Design review of the part built by this model. Coordinates are the model's own, in mm. Give positions to 0.01 mm unless a question says otherwise; leave off trailing zeros. Loops run counter-clockwise (first coordinate to the right, second up) from the corner with the lowest first, then second, coordinate; pieces in that order, holes last. Notation, with made-up numbers: (47, 82) -> (64, 82) arc R24 ccw to (64, 108) -> close; hole circle Ø1 at (62, 8.5). An arc over 180 degrees is marked (long way). Use CSV: the item, a comma, the result in double quotes. Start each with the question number.
Item 1: Clearance check with flat-ended pins moving along their axes: pin 1 (1.5 mm diameter, centred on x = 63.5, z = 22.5, fed in from -Y); pin 2 (1.5 mm diameter, centred on x = 85.5, y = 2, fed in from -Z); pin 3 (0.9 mm diameter, centred on x = -106.5, y = 1.5, fed in from +Z); pin 4 (1.5 mm diameter, centred on y = 1.5, z = -35.5, fed in from -X). State where each tip first meets the part, or that it passes through.
Item 2: We need section C-C (x = 70). State the section outline as (y, z) points, plus the area to 3 significant figures.
Item 3: We need section A-A (z = -1). State the section outline as (x, y) points, plus the area to 3 significant figures.
Item 4: We need section D-D (z = -32). State the section outline as (x, y) points.
Item 5: We need section B-B (y = 0.5). State the section outline as (x, z) points.
Item 6: Wall thickness on line 1 along X through (y, z) = (1.1, 10); line 2 along X through (y, z) = (1.15, 26); line 3 along Z through (x, y) = (3, 2.7): over which ranges is each line inside the solid? List them lowest first. Write a range as from..to.
from build123d import *

# Parameters (mm, degrees)
SKETCH1_W           = 3
SKETCH1_H           = 18
BOSS_EXTRUDE1_DEPTH = 3


with BuildPart() as part:
    # Sketch1 → Boss-Extrude1 (new body)
    with BuildSketch(Plane(origin=(0, 0, 0), x_dir=(1, 0, 0), z_dir=(0, 1, 0))):
        with BuildLine():
            Line((-100, 40), (-100, 25))
            Line((-100, 25), (-109, 25))
            Line((-109, 25), (-109, -25))
            Line((-109, -25), (-100, -25))
            Line((-100, -25), (-100, -40))
            ThreePointArc((-100, -40), (0, -57.157287525), (100, -40))
            Line((100, -40), (100, -25))
            Line((100, -25), (109, -25))
            Line((109, -25), (109, 25))
            Line((109, 25), (100, 25))
            Line((100, 25), (100, 40))
            ThreePointArc((100, 40), (0, 57.157287525), (-100, 40))
        make_face()
        with Locations((104.5, 0)):
            Rectangle(SKETCH1_W, SKETCH1_H, mode=Mode.SUBTRACT)
        with Locations((-104.5, 0)):
            Rectangle(SKETCH1_W, SKETCH1_H, mode=Mode.SUBTRACT)
        with BuildLine():
            Line((-72.5, -15), (-72.5, 15))
            ThreePointArc((-72.5, 15), (-70, 17.5), (-67.5, 15))
            Line((-67.5, 15), (-67.5, -15))
            ThreePointArc((-67.5, -15), (-70, -17.5), (-72.5, -15))
        make_face(mode=Mode.SUBTRACT)
        with BuildLine():
            Line((72.5, -15), (72.5, 15))
            ThreePointArc((72.5, 15), (70, 17.5), (67.5, 15))
            Line((67.5, 15), (67.5, -15))
            ThreePointArc((67.5, -15), (70, -17.5), (72.5, -15))
        make_face(mode=Mode.SUBTRACT)
    extrude(amount=BOSS_EXTRUDE1_DEPTH)


solid = part.part
Results found:
1,pin 1,"y = 0"
1,pin 2,"z = -44.94"
1,pin 3,"z = 25"
1,pin 4,"x = -100"
2,outline,"(0, -48.88) -> (3, -48.88) -> (3, -17.5) -> (0, -17.5) -> close; (0, 17.5) -> (3, 17.5) -> (3, 48.88) -> (0, 48.88) -> close"
2,area,"188 mm²"
3,outline,"(-109, 0) -> (-106, 0) -> (-106, 3) -> (-109, 3) -> close; (-103, 0) -> (-72.5, 0) -> (-72.5, 3) -> (-103, 3) -> close; (-67.5, 0) -> (67.5, 0) -> (67.5, 3) -> (-67.5, 3) -> close; (72.5, 0) -> (103, 0) -> (103, 3) -> (72.5, 3) -> close; (106, 0) -> (109, 0) -> (109, 3) -> (106, 3) -> close"
3,area,"606 mm²"
4,outline,"(-100, 0) -> (100, 0) -> (100, 3) -> (-100, 3) -> close"
5,outline,"(-109, -25) -> (-100, -25) -> (-100, -40) arc R300 ccw to (100, -40) -> (100, -25) -> (109, -25) -> (109, 25) -> (100, 25) -> (100, 40) arc R300 ccw to (-100, 40) -> (-100, 25) -> (-109, 25) -> close; hole (-106, -9) -> (-103, -9) -> (-103, 9) -> (-106, 9) -> close; hole (-72.5, -15) arc R2.5 ccw to (-67.5, -15) -> (-67.5, 15) arc R2.5 ccw to (-72.5, 15) -> close; hole (67.5, -15) arc R2.5 ccw to (72.5, -15) -> (72.5, 15) arc R2.5 ccw to (67.5, 15) -> close; hole (103, -9) -> (106, -9) -> (106, 9) -> (103, 9) -> close"
6,line 1,"-109..-72.5, -67.5..67.5, 72.5..109"
6,line 2,"-100..100"
6,line 3,"-57.14..57.14"
